The model under review builds one solid part; all positions refer to its coordinate system, in mm. A direction names the side the tool comes from. Coordinates: 2 decimals unless noted, no trailing zeros. Order: outer loops, then holes, each group sorted by start corner. A loop starts at its lowest first (then second) coordinate and runs counter-clockwise, first axis right, second up. Notation, with made-up numbers: (-23, -8.75) - (11, -8.75) arc R19 cw to (11, 5.25) - close; hole circle Ø8 at (-29, 49). An arc over 180 degrees is marked (long way). Answer in a Markdown table with one row per item.
```python
from build123d import *

# Parameters (mm, degrees)
F1_DEPTH = 15
F2_SIZE  = 0.5
F3_SIZE  = 2


with BuildPart() as f1:
    # F0 (on Top) → F1 (new body)
    with BuildSketch(Plane.XY):
        Polygon((0, 2), (0, 0), (20, 0), (20, -6), (12, -6), (12, -8), (20, -8), (22, -8), (22, -6), (22, 0), (22, 2), (20, 2), align=None)
    extrude(amount=F1_DEPTH)

    # F2
    f2_edges = [f1.edges().sort_by_distance(p)[0] for p in [
        (0, 2, 7.5),
        (0, 0, 7.5),
        (12, -8, 7.5),
        (12, -6, 7.5),
        (22, -8, 7.5),
        (22, 2, 7.5),
    ]]
    chamfer(f2_edges, length=F2_SIZE)

    # F3
    f3_edges = [f1.edges().sort_by_distance(p)[0] for p in [
        (20, 0, 7.5),
        (20, -6, 7.5),
    ]]
    chamfer(f3_edges, length=F3_SIZE)


solid = f1.part
```
Item 1: We need section A-A, the plane x = 13. Write out the cut boundary in (y, z).
Check values:
| item | result |
|---|---|
| outline | (-8, 0) - (-6, 0) - (-6, 15) - (-8, 15) - close; (0, 0) - (2, 0) - (2, 15) - (0, 15) - close |
Item 2: To check wall thickness, follow line 1 (Y direction, x = 13.5, z = 5.5); line 2 (Y direction, x = 8, z = 1); line 3 (X direction, y = -3, z = 13.25). State the ranges of each line that lie inside material, in increasing order. Write a range as from..to.
Check values:
| item | result |
|---|---|
| line 1 | -8..-6, 0..2 |
| line 2 | 0..2 |
| line 3 | 20..22 |
Item 3: Clearance check with flat-ended pins moving along their axes: pin 1 Ø0.8 at (y, z) = (-7, 4) entering from -X; pin 2 Ø3 at (x, y) = (14, -3) entering from +Z; pin 3 Ø3 at (x, z) = (6.5, 6) entering from -Y; pin 4 Ø1 at (y, z) = (-4, 10) entering from -X. State where each tip first meets the part, or that it passes through.
Check values:
| item | result |
|---|---|
| pin 1 | x = 12 |
| pin 2 | through |
| pin 3 | y = 0 |
| pin 4 | x = 19.5 |
Item 4: We need section B-B, the plane z = 13. Write out the cut boundary in (x, y), then the cut area to 4 significant figures.
Check values:
| item | result |
|---|---|
| outline | (0, 0.5) - (0.5, 0) - (18, 0) - (20, -2) - (20, -4) - (18, -6) - (12.5, -6) - (12, -6.5) - (12, -7.5) - (12.5, -8) - (21.5, -8) - (22, -7.5) - (22, 1.5) - (21.5, 2) - (0.5, 2) - (0, 1.5) - close |
| area | 79.25 mm^2 |
Item 5: Tool access review of faces 1 (the face through (17, -8, 7)), 2 (the face through (12, -7, 7)), 3 (the face through (9, 0, 7)): name each direction out of +Z, -Z, +X, -X, +Y, -Y from which nothing blocks a thin tool from reaching the whole face with its end or side.
Check values:
| item | result |
|---|---|
| face 1 | +Z, -Z, +X, -X, -Y |
| face 2 | +Z, -Z, -X, -Y |
| face 3 | +Z, -Z, -X |
Item 6: We need section C-C, the plane y = -2.5. Write out the cut boundary in (x, z), then the cut area to 3 significant figures.
Check values:
| item | result |
|---|---|
| outline | (20, 0) - (22, 0) - (22, 15) - (20, 15) - close |
| area | 30.0 mm^2 |
Item 7: Mouldability with a two-part tool opening along Y and no side actions: class faces 4 (the face through (11, 2, 7)), 5 (the face through (0, 1, 7)), 6 (the face through (15, -6, 7)), 7 (the face through (20, -3, 7)) as +Y half, -Y half, draft (parallel to the pull), parting line (faces both ways), or undercut.
Check values:
| item | result |
|---|---|
| face 4 | +Y half |
| face 5 | draft |
| face 6 | undercut |
| face 7 | undercut |
Item 8: We need section D-D, the plane x = 8. Write out the cut boundary in (y, z).
Check values:
| item | result |
|---|---|
| outline | (0, 0) - (2, 0) - (2, 15) - (0, 15) - close |
